Can you work these out from the drawing? Everything is in mm from the part's minimum corner. A direction names the side the tool comes from. Coordinates: 2 decimals unless noted, no trailing zeros. Loops run counter-clockwise (first coordinate to the right, second up) from the corner with the lowest first, then second, coordinate; pieces in that order, holes last.
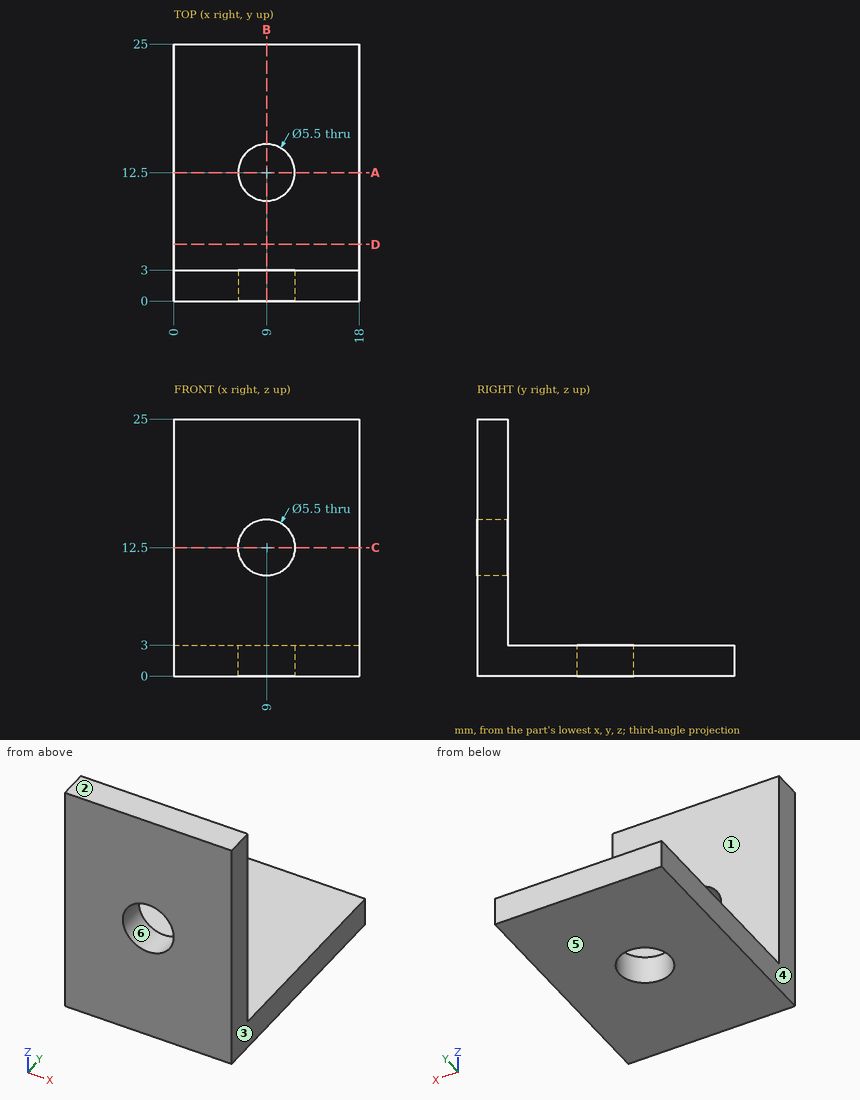
Item 1: I need wall thicknesses on line 1 along Y through (x, z) = (9, 2.45); line 2 along X through (y, z) = (2.2, 12.5); line 3 along Z through (x, y) = (10.25, 4.75). Which ranges of each line are inside material? Lowest first, please.
Results are:
line 1: y = 0 to 9.75, 15.25 to 25
line 2: x = 0 to 6.25, 11.75 to 18
line 3: z = 0 to 3
Item 2: On a 3-axis mill with a long thin cutter (end or side, diameter ignored), from which of +Z, -Z, +X, -X, +Y, -Y can I reach the whole of each face in a straight line? I mean the marked faces 1 and 2. Say none if no direction works.
Results are:
face 1: +Z, +X, -X, +Y
face 2: +Z, +X, -X, +Y, -Y
Item 3: Suppose I cut it at A-A, the plane y = 12.5. Please give me the cut outline in (x, z), plus the area to 3 significant figures.
Results are:
outline: (0, 0) - (6.25, 0) - (6.25, 3) - (0, 3) - close; (11.75, 0) - (18, 0) - (18, 3) - (11.75, 3) - close
area: 37.5 mm2
Item 4: I'm going to push flat-ended pins straight in: P1, Ø5, axis at x = 2, z = 20.5, coming from the +Y side; P2, Ø9, axis at x = 13.5, y = 18.5, coming from the +Z side. Where does each tip first touch, or does it pass through?
Results are:
P1: stops at y = 3
P2: stops at z = 3
Item 5: Suppose I cut it at B-B, the plane x = 9. Please give me the cut outline in (y, z).
Results are:
outline: (0, 0) - (9.75, 0) - (9.75, 3) - (3, 3) - (3, 9.75) - (0, 9.75) - close; (0, 15.25) - (3, 15.25) - (3, 25) - (0, 25) - close; (15.25, 0) - (25, 0) - (25, 3) - (15.25, 3) - close
Item 6: Suppose I cut it at D-D, the plane y = 5.5. Please give me the cut outline in (x, z).
Results are:
outline: (0, 0) - (18, 0) - (18, 3) - (0, 3) - close
Item 7: We'd pull the mould along X, two halves only. Please class the marked faces 3, 4, 5 and 6: +X half, -X half, draft (parallel to the pull), parting line (faces both ways), or undercut.
Results are:
face 3: +X half
face 4: -X half
face 5: draft
face 6: undercut
